Work out the finished part from the listing and answer in its coordinate system (mm). Face numbers are marked on the shaded views. Round coordinates to 2 decimals unless told otherwise and drop trailing zeros. Order: outer loops, then holes, each group sorted by start corner. A loop starts at its lowest first (then second) coordinate and runs counter-clockwise, first axis right, second up. Notation, with made-up numbers: (-32.5, 9) - (-25.5, 9) arc R6 cw to (-25.5, 18) - close; hole circle Ø10 at (-22, 13.5). An arc over 180 degrees is marked (long way). Use one line per item in the form item = value. Start each with the question number.
Q1. The part is cut by section A-A on x = 0. Determine the outline of the cut face in (y, z).
Q2. The part is cut by section C-C on x = 7.5. Determine the outline of the cut face in (y, z), plus the area to 3 significant figures.
Q3. The part is cut by section D-D on z = 2.5. Determine the outline of the cut face in (x, y).
Q4. Find the intervals of material crossed by line 1 (X direction, y = -5, z = 1.25); line 2 (Z direction, x = -7.5, y = -10.2); line 3 (X direction, y = 18, z = 0), in increasing order. Write a range as [from, to].
Q5. The part is cut by section B-B on z = -1. Determine the outline of the cut face in (x, y), plus the area to 3 significant figures.
Q6. For a pull along Y with two mould halves and no side action, classify the marked faces 1, 2, 3 and 4 as +Y half, -Y half, draft (parallel to the pull), parting line (faces both ways), or undercut.
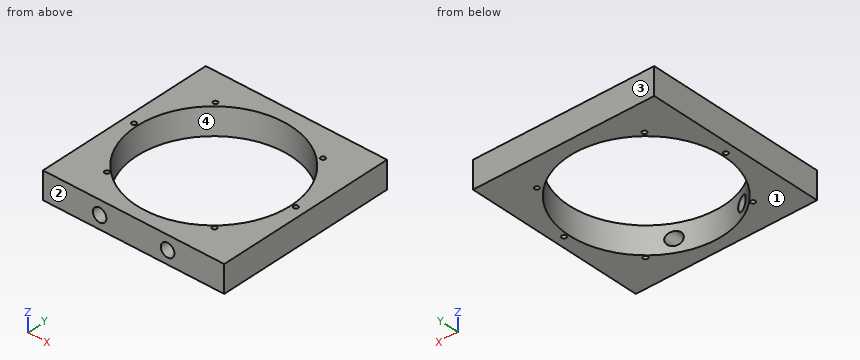
from build123d import *

# Parameters (mm, degrees)
SKETCH1_W           = 40
SKETCH1_H           = 40
BOSS_EXTRUDE1_DEPTH = 3
SKETCH3_R           = 0.5
CUT_EXTRUDE1_DEPTH  = 40
SKETCH4_R           = 1.5
CUT_EXTRUDE3_DEPTH  = 30
SKETCH5_R           = 17
CUT_EXTRUDE7_DEPTH  = 36.186486738


with BuildPart() as part:
    # Sketch1 → Boss-Extrude1 (new, symmetric)
    with BuildSketch(Plane.XY):
        with Locations((0, 8.321173156)):
            Rectangle(SKETCH1_W, SKETCH1_H)
    extrude(amount=BOSS_EXTRUDE1_DEPTH, both=True)

    # Sketch3 → Cut-Extrude1 (cut)
    with BuildSketch(Plane.XY.offset(3)):
        with Locations((-11.872178248, 21.659280154)):
            Circle(SKETCH3_R)
        with Locations((-17.856475427, 8.321173156)):
            Circle(SKETCH3_R)
        with Locations((-11.872178248, -5.016933842)):
            Circle(SKETCH3_R)
        with Locations(Location((11.872178248, -5.016933842, 0), (0, 0, 180))):
            Circle(SKETCH3_R)
        with Locations(Location((17.856475427, 8.321173156, 0), (0, 0, 180))):
            Circle(SKETCH3_R)
        with Locations(Location((11.872178248, 21.659280154, 0), (0, 0, 180))):
            Circle(SKETCH3_R)
    extrude(amount=-CUT_EXTRUDE1_DEPTH, mode=Mode.SUBTRACT)

    # Sketch4 → Cut-Extrude3 (cut)
    with BuildSketch(Plane(origin=(0, 0, 0), x_dir=(1, 0, 0), z_dir=(0, 1, 0))):
        with Locations(Location((-7.5, 0.085145046, 0), (0, 0, 270))):
            Circle(SKETCH4_R)
        with Locations(Location((7.5, 0.085145046, 0), (0, 0, 270))):
            Circle(SKETCH4_R)
    extrude(amount=-CUT_EXTRUDE3_DEPTH, mode=Mode.SUBTRACT)

    # Sketch5 → Cut-Extrude7 (cut, through all)
    with BuildSketch(Plane.XY.offset(3)):
        with Locations((0, 8.01211428)):
            Circle(SKETCH5_R)
    extrude(amount=-CUT_EXTRUDE7_DEPTH, mode=Mode.SUBTRACT)


solid = part.part
Found:
q1.outline = (-11.68, -3) - (-8.99, -3) - (-8.99, 3) - (-11.68, 3) - close; (25.01, -3) - (28.32, -3) - (28.32, 3) - (25.01, 3) - close
q2.outline = (-11.68, -3) - (-7.24, -3) - (-7.24, -1.59) - (-11.68, -1.59) - close; (-11.68, 1.41) - (-7.24, 1.41) - (-7.24, 3) - (-11.68, 3) - close; (23.27, -3) - (28.32, -3) - (28.32, 3) - (23.27, 3) - close
q2.area = 43.6 mm²
q3.outline = (-20, -11.68) - (20, -11.68) - (20, 28.32) - (-20, 28.32) - close; hole circle Ø1 at (-17.86, 8.32); hole circle Ø34 at (0, 8.01); hole circle Ø1 at (-11.87, -5.02); hole circle Ø1 at (-11.87, 21.66); hole circle Ø1 at (11.87, -5.02); hole circle Ø1 at (11.87, 21.66); hole circle Ø1 at (17.86, 8.32)
q4.line_1 = [-20, -12.37], [-11.37, -10.94], [10.94, 11.37], [12.37, 20]
q4.line_2 = [-3, -1.59], [1.41, 3]
q4.line_3 = [-20, -13.76], [13.76, 20]
q5.outline = (-20, -11.68) - (-8.69, -11.68) - (-8.69, -6.6) arc R17 cw (long way) to (8.69, -6.6) - (8.69, -11.68) - (20, -11.68) - (20, 28.32) - (-20, 28.32) - close; (-6.31, -11.68) - (6.31, -11.68) - (6.31, -7.77) arc R17 cw to (-6.31, -7.77) - close; hole circle Ø1 at (-17.86, 8.32); hole circle Ø1 at (-11.87, -5.02); hole circle Ø1 at (-11.87, 21.66); hole circle Ø1 at (11.87, -5.02); hole circle Ø1 at (11.87, 21.66); hole circle Ø1 at (17.86, 8.32)
q5.area = 666 mm²
q6.face_1 = draft
q6.face_2 = -Y half
q6.face_3 = +Y half
q6.face_4 = undercut
